CAD build for the part. Positions are in the model's coordinates, mm. Coordinates: 2 decimals unless noted, no trailing zeros. Write each loop counter-clockwise with the first axis right and the second up, starting at its lowest first coordinate (ties: lowest second). Pieces come first, ordered by that corner, then holes. Notation, with made-up numbers: M 75.5,25.25 L 92.5,25.25 A23 cw 92.5,37.25 Z; hole C -4.75,-33 d7. An arc over 180 degrees is marked long. Put each result on its own line as item: value. Start each with the question number.
```python
from build123d import *

# Parameters (mm, degrees)
SKETCH1_W           = 176
SKETCH1_H           = 41
SKETCH1_R           = 4.5
BOSS_EXTRUDE1_DEPTH = 3
FILLET1_R           = 1


with BuildPart() as part:
    # Sketch1 → Boss-Extrude1 (new, symmetric)
    with BuildSketch(Plane.XY):
        with Locations((88, 20.5)):
            Rectangle(SKETCH1_W, SKETCH1_H)
        with Locations((20.5, 20.5)):
            Circle(SKETCH1_R, mode=Mode.SUBTRACT)
        with Locations((65.5, 20.5)):
            Circle(SKETCH1_R, mode=Mode.SUBTRACT)
        with Locations((110.5, 20.5)):
            Circle(SKETCH1_R, mode=Mode.SUBTRACT)
        with Locations((155.5, 20.5)):
            Circle(SKETCH1_R, mode=Mode.SUBTRACT)
    extrude(amount=BOSS_EXTRUDE1_DEPTH, both=True)

    # Fillet1
    fillet1_edges = [part.edges().sort_by_distance(p)[0] for p in [
        (88, 41, 3),
        (0, 20.5, 3),
        (88, 0, 3),
        (176, 20.5, 3),
        (0, 0, 0),
        (0, 41, 0),
        (176, 41, 0),
        (176, 0, 0),
    ]]
    fillet(fillet1_edges, radius=FILLET1_R)


solid = part.part
```
(1) Slice it at C-C, the plane z = 0.4. Write the cut outline in (x, y).
(2) Slice it at B-B, the plane y = 20.5. Write the cut outline in (x, z).
(3) Slice it at A-A, the plane x = 20.5. Write the cut outline in (y, z), then the cut area to 3 significant figures.
(4) Drill centre lines: line 1 (Y direction, x = 110.5, z = -0.2); line 2 (Y direction, x = 158, z = 0.15); line 3 (X direction, y = 26.5, z = 2.6). Where is each one in solid material? Low to high. Write a range as [from, to].
(5) Two-plate mould, pull along X, no slides. Class faces 1 (the face through (106.004, 20.698, -0.042)), 2 (the face through (176, 20, 0)), 3 (the face through (87, 21, -3)): +X half, -X half, draft (parallel to the pull), parting line (faces both ways), or undercut.
(6) Slice it at D-D, the plane x = 112. Write the cut outline in (y, z), then the cut area to 3 significant figures.
Result set:
1. outline: M 0,1 A1 ccw 1,0 L 175,0 A1 ccw 176,1 L 176,40 A1 ccw 175,41 L 1,41 A1 ccw 0,40 Z; hole C 20.5,20.5 d9; hole C 65.5,20.5 d9; hole C 110.5,20.5 d9; hole C 155.5,20.5 d9
2. outline: M 0,-3 L 16,-3 L 16,3 L 1,3 A1 ccw 0,2 Z; M 25,-3 L 61,-3 L 61,3 L 25,3 Z; M 70,-3 L 106,-3 L 106,3 L 70,3 Z; M 115,-3 L 151,-3 L 151,3 L 115,3 Z; M 160,-3 L 176,-3 L 176,2 A1 ccw 175,3 L 160,3 Z
3. outline: M 0,-3 L 16,-3 L 16,3 L 1,3 A1 ccw 0,2 Z; M 25,-3 L 41,-3 L 41,2 A1 ccw 40,3 L 25,3 Z
3. area: 192 mm^2
4. line 1: y = [0, 16], [25, 41]
4. line 2: y = [0, 16.76], [24.24, 41]
4. line 3: x = [0.2, 175.8]
5. face 1: undercut
5. face 2: +X half
5. face 3: draft
6. outline: M 0,-3 L 16.26,-3 L 16.26,3 L 1,3 A1 ccw 0,2 Z; M 24.74,-3 L 41,-3 L 41,2 A1 ccw 40,3 L 24.74,3 Z
6. area: 195 mm^2
